Read the model definition and answer for the solid it produces. Units are mm, in the model's axes. A direction names the side the tool comes from. Coordinates: 2 decimals unless noted, no trailing zeros. Order: outer loops, then holes, each group sorted by start corner. A loop starts at its lowest first (then second) coordinate and runs counter-clockwise, first axis right, second up. Notation, with made-up numbers: (86, 46) - (99, 46) arc R21 cw to (99, 60) - close; hole circle Ø9 at (63.25, -19). An arc over 180 degrees is marked (long way). Use one line per item in the form item = value.
```python
from build123d import *

# Parameters (mm, degrees)
SKETCH2_R                    = 17
BOSS_EXTRUDE1_DEPTH          = 29
SKETCH3_R                    = 12.5
BOSS_EXTRUDE2_DEPTH          = 11
CUT_EXTRUDE1_DEPTH           = 1.5
F_3_0_3_DIAMETER_HOLE1_D     = 3
F_3_0_3_DIAMETER_HOLE1_DEPTH = 3
CHAMFER1_SIZE                = 0.5


with BuildPart() as part:
    # Sketch1 → Revolve1 (revolve)
    with BuildSketch(Plane.XZ, mode=Mode.PRIVATE) as revolve1_sk:
        with BuildLine():
            Line((18.4, 52), (0, 52))
            Line((0, 52), (0, 29))
            Line((0, 29), (17, 29))
            ThreePointArc((17, 29), (16.707106781, 29.707106781), (16, 30))
            Line((16, 30), (18.4, 30))
            Line((18.4, 30), (18.4, 52))
        make_face()
    revolve(revolve1_sk.sketch.rotate(Axis((0, 0, 52), (0, 0, -1)), 180), axis=Axis((0, 0, 52), (0, 0, -1)))

    # Sketch2 → Boss-Extrude1 (add)
    with BuildSketch(Plane(origin=(0, 0, 29), x_dir=(-1, 0, 0), z_dir=(0, 0, -1))):
        Circle(SKETCH2_R)
    extrude(amount=BOSS_EXTRUDE1_DEPTH)

    # Sketch3 → Boss-Extrude2 (add)
    with BuildSketch(Plane(origin=(0, 0, 0), x_dir=(-1, 0, 0), z_dir=(0, 0, -1))):
        Circle(SKETCH3_R)
    extrude(amount=BOSS_EXTRUDE2_DEPTH)

    # Sketch4 → Cut-Extrude1 (cut)
    with BuildSketch(Plane.XY.offset(52)):
        with BuildLine():
            ThreePointArc((8.868134735, 8.359715213), (-12.187233161, 0), (8.868134735, -8.359715213))
            ThreePointArc((8.868134735, -8.359715213), (-1.565907181, 0), (8.868134735, 8.359715213))
        make_face()
    extrude(amount=-CUT_EXTRUDE1_DEPTH, mode=Mode.SUBTRACT)

    # Sketch5 → Revolve2 (revolve)
    with BuildSketch(Plane.XZ, mode=Mode.PRIVATE) as revolve2_sk:
        Polygon((10, 74), (7, 74), (7, 52), (13, 52), (13, 58.5), (10, 58.5), align=None)
    revolve(revolve2_sk.sketch.rotate(Axis((7, 0, 74), (0, 0, -1)), 180), axis=Axis((7, 0, 74), (0, 0, -1)))

    # Ø3.0 (3) Diameter Hole1
    with Locations(Plane.XY.offset(52)):
        with Locations((-13.423393759, 7.75), (-13.423393759, -7.75), (0, -15.5), (13.423393759, -7.75), (13.423393759, 7.75), (0, 15.5)):
            Hole(F_3_0_3_DIAMETER_HOLE1_D / 2, depth=F_3_0_3_DIAMETER_HOLE1_DEPTH)

    # Chamfer1
    chamfer1_edges = [part.edges().sort_by_distance(p)[0] for p in [
        (13, 0, 58.5),
    ]]
    chamfer(chamfer1_edges, length=CHAMFER1_SIZE)


solid = part.part
```
(1) Section D-D, the plane z = 4 is taken. Write down the section's boundary in (x, y), then the cut area to 3 significant figures.
Answer list:
outline = circle Ø34 at (0, 0)
area = 908 mm2
(2) Which of the six approach directions +Z, -Z, +X, -X, +Y, -Y give full straight-line access (tool end or side, diameter ignored) to faces 1 (the cylindrical face through (13.749, -9.214, 50.479)), 2 (the cylindrical face through (-11.923, 3.755, -5.423)), 3 (the flat face through (0, 0, -11))?
Answer list:
face_1 = +Z
face_2 = -Z
face_3 = -Z, +X, -X, +Y, -Y
(3) Straight lines are drawn through the part: L1, parallel to Y at x = 0, z = 50; L2, parallel to X at y = 7, z = 50; L3, parallel to Y at x = 0, z = 51.5. For each, find the intervals that lie inside material, in ascending order.
Answer list:
L1 = -18.4 to -17, -14 to 14, 17 to 18.4
L2 = -17.02 to -14.72, -12.12 to 12.12, 14.72 to 17.02
L3 = -18.4 to -17, -14 to -12.19, -4.94 to 4.94, 12.19 to 14, 17 to 18.4
(4) Given pin 1 Ø10 at (y, z) = (-4.5, 6.5) entering from +X; pin 2 Ø3.5 at (x, y) = (-13, 7.5) entering from +Z; pin 3 Ø5 at (x, y) = (13.42, 7.75) entering from -Z; pin 4 Ø11 at (x, y) = (7, 6.5) entering from +Z, each flat-ended and moving along its own axis, determine where each tip first touches the part or whether it passes through.
Answer list:
pin_1 = 17
pin_2 = 52
pin_3 = 0
pin_4 = 74
(5) Section B-B, the plane z = 36 is taken. Write down the section's boundary in (x, y), then the cut area to 3 significant figures.
Answer list:
outline = circle Ø36.8 at (0, 0)
area = 1,060 mm2
(6) Section A-A, the plane y = 0 is taken. Write down the section's boundary in (x, z).
Answer list:
outline = (-18.4, 30) - (-16, 30) arc R1 ccw to (-17, 29) - (-17, 0) - (-12.5, 0) - (-12.5, -11) - (12.5, -11) - (12.5, 0) - (17, 0) - (17, 29) arc R1 ccw to (16, 30) - (18.4, 30) - (18.4, 52) - (13, 52) - (13, 58) - (12.5, 58.5) - (10, 58.5) - (10, 74) - (4, 74) - (4, 58.5) - (1.5, 58.5) - (1, 58) - (1, 52) - (-1.57, 52) - (-1.57, 50.5) - (-12.19, 50.5) - (-12.19, 52) - (-18.4, 52) - close
(7) The mould has two halves that part along X. Classify faces 4 (the cylindrical face through (-9.139, 14.334, 14.703)), 5 (the flat face through (0, 0, 52)), 6 (the cylindrical face through (0, -17, 50)): +X half, -X half, draft (parallel to the pull), parting line (faces both ways), or undercut.
Answer list:
face_4 = parting line
face_5 = draft
face_6 = undercut
